from build123d import *

# Parameters (mm, degrees)
SKETCH1_W           = 107.7
SKETCH1_H           = 47.7
BOSS_EXTRUDE1_DEPTH = 6.35


with BuildPart() as part:
    # Sketch1 → Boss-Extrude1 (new body)
    with BuildSketch(Plane.XY):
        with Locations((0, 23.85)):
            Rectangle(SKETCH1_W, SKETCH1_H)
        with BuildLine():
            Line((34.500012, 7.8), (-34.499988, 7.8))
            ThreePointArc((-34.499988, 7.8), (-35.914201562, 8.385786438), (-36.499988, 9.8))
            Line((-36.499988, 9.8), (-36.499988, 35.2))
            ThreePointArc((-36.499988, 35.2), (-35.914201562, 36.614213562), (-34.499988, 37.2))
            Line((-34.499988, 37.2), (34.500012, 37.2))
            ThreePointArc((34.500012, 37.2), (35.914225562, 36.614213562), (36.500012, 35.2))
            Line((36.500012, 35.2), (36.500012, 9.8))
            ThreePointArc((36.500012, 9.8), (35.914225562, 8.385786438), (34.500012, 7.8))
        make_face(mode=Mode.SUBTRACT)
    extrude(amount=BOSS_EXTRUDE1_DEPTH)


solid = part.part
For this review, take the finished solid that the model builds, in its own axes (mm). A direction names the side the tool comes from. Give positions to 0.01 mm unless a question says otherwise; leave off trailing zeros. Write each loop counter-clockwise with the first axis right and the second up, starting at its lowest first coordinate (ties: lowest second). Pieces come first, ordered by that corner, then holes. Notation, with made-up numbers: (-29, -19.5) -> (13, -19.5) arc R9 cw to (13, -15.5) -> close; hole circle Ø10 at (23, 26.5). An arc over 180 degrees is marked (long way). Use CSV: the item, a comma, the result in double quotes.
Q1. To check wall thickness, follow probe 1 along Y at (x, z) = (-22, 6); probe 2 along X at (y, z) = (19, 1.25); probe 3 along Y at (x, z) = (-35, 5.25). State the ranges of each line that lie inside material, in increasing order. Write a range as [from, to].
Conclusion:
probe 1,"[0, 7.8], [37.2, 47.7]"
probe 2,"[-53.85, -36.5], [36.5, 53.85]"
probe 3,"[0, 7.86], [37.14, 47.7]"
Q2. Take a section at A-A, the plane y = 24. Write out the cut boundary in (x, z).
Conclusion:
outline,"(-53.85, 0) -> (-36.5, 0) -> (-36.5, 6.35) -> (-53.85, 6.35) -> close; (36.5, 0) -> (53.85, 0) -> (53.85, 6.35) -> (36.5, 6.35) -> close"
Q3. Tool access review of faces 4 (the face through (-35.9, 8.37, 3.13)), 5 (the face through (-1, 40, 6.35)): name each direction out of +Z, -Z, +X, -X, +Y, -Y from which nothing blocks a thin tool from reaching the whole face with its end or side.
Conclusion:
face 4,"+Z, -Z"
face 5,"+Z, +X, -X, +Y, -Y"
Q4. Take a section at B-B, the plane x = 8. Write out the cut boundary in (y, z).
Conclusion:
outline,"(0, 0) -> (7.8, 0) -> (7.8, 6.35) -> (0, 6.35) -> close; (37.2, 0) -> (47.7, 0) -> (47.7, 6.35) -> (37.2, 6.35) -> close"
Q5. Mouldability with a two-part tool opening along Y and no side actions: class faces 1 (the face through (-1, 0, 3)), 2 (the face through (0, 7.8, 3)), 3 (the face through (53.85, 24, 3)) as pulls with the +Y half, pulls with the -Y half, needs draft (parallel to the pull), parting line crosses it, or undercut.
Conclusion:
face 1,"pulls with the -Y half"
face 2,"undercut"
face 3,"needs draft"
Q6. Take a section at C-C, the plane z = 3.5. Write out the cut boundary in (x, y), then the cut area to 3 significant figures.
Conclusion:
outline,"(-53.85, 0) -> (53.85, 0) -> (53.85, 47.7) -> (-53.85, 47.7) -> close; hole (-36.5, 9.8) arc R2 ccw to (-34.5, 7.8) -> (34.5, 7.8) arc R2 ccw to (36.5, 9.8) -> (36.5, 35.2) arc R2 ccw to (34.5, 37.2) -> (-34.5, 37.2) arc R2 ccw to (-36.5, 35.2) -> close"
area,"2,990 mm2"
